CAD build for the part. Positions are in the model's coordinates, mm. A direction names the side the tool comes from. Give positions to 0.01 mm unless a question says otherwise; leave off trailing zeros. Order: outer loops, then holes, each group sorted by start corner. A loop starts at its lowest first (then second) coordinate and runs counter-clockwise, first axis right, second up. Notation, with made-up numbers: (41, 9.25) -> (89, 9.25) arc R22 cw to (89, 26.25) -> close; hole circle Ø9 at (81.5, 54.5). An arc over 180 degrees is marked (long way). Answer as CSV lines item,"result".
```python
from build123d import *

# Parameters (mm, degrees)
SKETCH1_R               = 9
BOSS_EXTRUDE1_DEPTH     = 8
SKETCH3_R               = 11
BOSS_EXTRUDE2_DEPTH     = 3
SKETCH4_R               = 11
BOSS_EXTRUDE3_DEPTH     = 3
SKETCH2_R               = 3
CUT_EXTRUDE1_DEPTH      = 3
CUT_EXTRUDE1_DEPTH_BACK = 11


with BuildPart() as part:
    # Sketch1 → Boss-Extrude1 (new body)
    with BuildSketch(Plane(origin=(0, 0, 0), x_dir=(0, 0, -1), z_dir=(1, 0, 0))):
        Circle(SKETCH1_R)
    extrude(amount=BOSS_EXTRUDE1_DEPTH)

    # Sketch3 → Boss-Extrude2 (add)
    with BuildSketch(Plane(origin=(8, 0, 0), x_dir=(0, 0, -1), z_dir=(1, 0, 0))):
        Circle(SKETCH3_R)
    extrude(amount=BOSS_EXTRUDE2_DEPTH)

    # Sketch4 → Boss-Extrude3 (add)
    with BuildSketch(Plane.ZY):
        Circle(SKETCH4_R)
    extrude(amount=BOSS_EXTRUDE3_DEPTH)

    # Sketch2 → Cut-Extrude1 (cut, two sides)
    with BuildSketch(Plane(origin=(8, 0, 0), x_dir=(0, 0, -1), z_dir=(1, 0, 0))) as cut_extrude1_sk:
        Circle(SKETCH2_R)
    extrude(amount=CUT_EXTRUDE1_DEPTH, mode=Mode.SUBTRACT)
    extrude(cut_extrude1_sk.sketch, amount=-CUT_EXTRUDE1_DEPTH_BACK, mode=Mode.SUBTRACT)


solid = part.part
```
1) Wall check: line 1 along Y through (x, z) = (5, 0); line 2 along X through (y, z) = (-9.25, -3.5); line 3 along Y through (x, z) = (9.4, 0). Give the ranges that are in metal, low to high. Write a range as [from, to].
Data:
line 1,"y = [-9, -3], [3, 9]"
line 2,"x = [-3, 0], [8, 11]"
line 3,"y = [-11, -3], [3, 11]"
2) Band-saw the part on C-C, the plane x = 4. Write the cut outline in (y, z).
Data:
outline,"circle Ø18 at (0, 0); hole circle Ø6 at (0, 0)"
3) Band-saw the part on A-A, the plane z = 0. Write the cut outline in (x, y), then the cut area to 3 significant figures.
Data:
outline,"(-3, -11) -> (0, -11) -> (0, -9) -> (8, -9) -> (8, -11) -> (11, -11) -> (11, -3) -> (-3, -3) -> close; (-3, 3) -> (11, 3) -> (11, 11) -> (8, 11) -> (8, 9) -> (0, 9) -> (0, 11) -> (-3, 11) -> close"
area,"192 mm2"
4) Which spindle directions (+Z, -Z, +X, -X, +Y, -Y) get a long thin tool onto all of the face, cutting with end or side? Do faces 1 (the flat face through (11, -2.3, -2.3)), 2 (the flat face through (8, -9, -2)). Say none if no direction does.
Data:
face 1,"+Z, -Z, +X, +Y, -Y"
face 2,"none"
5) Band-saw the part on D-D, the plane y = -3.5. Write the cut outline in (x, z), then the cut area to 3 significant figures.
Data:
outline,"(-3, -10.43) -> (0, -10.43) -> (0, -8.29) -> (8, -8.29) -> (8, -10.43) -> (11, -10.43) -> (11, 10.43) -> (8, 10.43) -> (8, 8.29) -> (0, 8.29) -> (0, 10.43) -> (-3, 10.43) -> close"
area,"258 mm2"
6) Pin check, flat tips, straight feed: P1, Ø1, axis at x = 6, z = 7.5, coming from the -Y side; P2, Ø6, axis at x = 8, y = -2, coming from the +Z side; P3, Ø5.5, axis at y = 0, z = 0, coming from the +X side; P4, Ø1.5, axis at x = 7.5, y = 6, coming from the -Z side. Stop position of each tip, or through.
Data:
P1,"stops at y = -5.66"
P2,"stops at z = 11"
P3,"passes through"
P4,"stops at z = -9.56"
7) Pull direction X, two halves, no side cores. Call faces 3 (the flat face through (-3, -2.3, 2.3)), 4 (the flat face through (0, -9, 2)), 5 (the cylindrical face through (9.48, -10.74, 2.38)): pulls with the +X half, pulls with the -X half, needs draft (parallel to the pull), parting line crosses it, or undercut.
Data:
face 3,"pulls with the -X half"
face 4,"undercut"
face 5,"needs draft"
